Geometry: see drawing. Coordinates: mm, zero at the bounding-box minimum. A direction names the side the tool comes from. Give positions to 0.01 mm unless a question says otherwise; leave off trailing zeros. Write each loop counter-clockwise with the first axis right and the second up, starting at its lowest first coordinate (ties: lowest second). Pieces come first, ordered by that corner, then holes. Notation, with made-up numbers: M 56,58.25 L 80,58.25 A33 cw 80,89.25 Z; hole C 74.5,-14.75 d4. An arc over 180 degrees is marked long. Use a Markdown table: item, result. Add a question column.
(1) Material intervals for L1, parallel to Y at x = 3, z = 11.25; L2, parallel to Y at x = 32.5, z = 11.5; L3, parallel to Y at x = 4, z = 13.75, sorted ascending.
(2) Cut plane D-D (z = 3.5). Output: boundary loops of the cut face in (x, y), plus the area to 3 significant figures.
(3) Draft query along X for the marked faces 1, 2 and 3. Return one class per face: released by +X, released by -X, zero draft, split by the parting line, or undercut.
(4) Cut plane C-C (x = 32). Output: boundary loops of the cut face in (y, z).
(5) Reachability of the marked faces 4 and 5 from +Z, -Z, +X, -X, +Y, -Y: full face, straight path, thin tool, end or side. Return the list, or none.
(6) Cut plane A-A (z = 9). State how many separate pieces and enclosed holes the cut face has, plus the area to 3 significant figures.
(7) Pin query (flat end, axial travel): pin 1 Ø1.5 at (x, y) = (56.5, 3) entering from +Z; pin 2 Ø1.2 at (y, z) = (20.475, 9) entering from +X (3 decimals). Return the tip coordinate at first contact, or that it passes through.
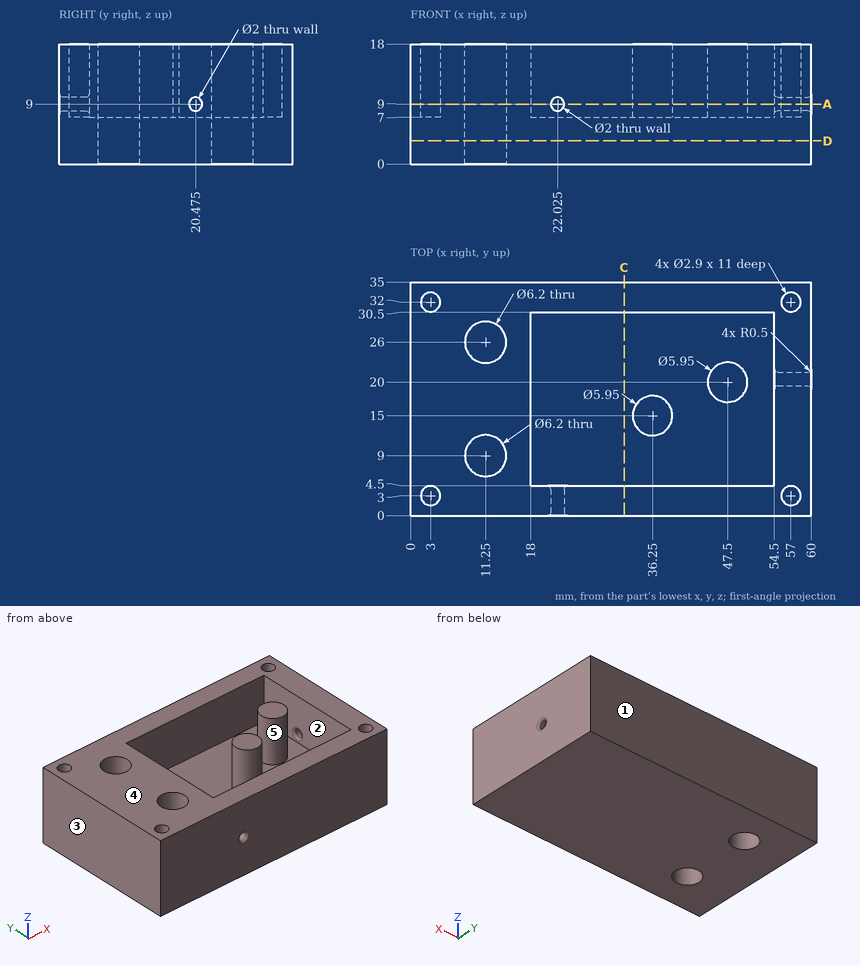
Answer list:
| question | item | result |
|---|---|---|
| 1 | L1 | 0 to 1.55, 4.45 to 30.55, 33.45 to 35 |
| 1 | L2 | 0 to 4.5, 30.5 to 35 |
| 1 | L3 | 0 to 1.95, 4.05 to 30.95, 33.05 to 35 |
| 2 | outline | M 0,0 L 60,0 L 60,35 L 0,35 Z; hole C 11.25,9 d6.2; hole C 11.25,26 d6.2 |
| 2 | area | 2,040 mm² |
| 3 | face 1 | zero draft |
| 3 | face 2 | undercut |
| 3 | face 3 | released by -X |
| 4 | outline | M 0,0 L 35,0 L 35,18 L 30.5,18 L 30.5,7 L 4.5,7 L 4.5,18 L 0,18 Z |
| 5 | face 4 | +Z, +X, -X, +Y, -Y |
| 5 | face 5 | +Z |
| 6 | separate pieces | 4 |
| 6 | enclosed holes | 6 |
| 6 | area | 1,100 mm² |
| 7 | pin 1 | z = 7 |
| 7 | pin 2 | x = 50.475 |
